```python
from build123d import *

# Parameters (mm, degrees)
F0_W     = 9.45931
F0_H     = 54.78517
F0_R     = 2.258507
F1_DEPTH = 0.4318
F0_R_2   = 1.35948
F2_DEPTH = 0.4064
F0_R_3   = 0.729172
F3_DEPTH = 0.3556
F4_DEPTH = 0.254


with BuildPart() as f1:
    # F0 (on Top) → F1 (new body, symmetric)
    with BuildSketch(Plane.XY):
        Rectangle(F0_W, F0_H)
        with Locations((0, -24.156982)):
            Circle(F0_R, mode=Mode.SUBTRACT)
    extrude(amount=F1_DEPTH, both=True)

    # F0 (on Top) → F2 (join)
    with BuildSketch(Plane.XY):
        with Locations((0, -24.156982)):
            Circle(F0_R)
        with Locations((0, -24.156982)):
            Circle(F0_R_2, mode=Mode.SUBTRACT)
    extrude(amount=F2_DEPTH)

    # F0 (on Top) → F3 (join)
    with BuildSketch(Plane.XY):
        with Locations((0, -24.156982)):
            Circle(F0_R_2)
        with Locations((0, -24.156982)):
            Circle(F0_R_3, mode=Mode.SUBTRACT)
    extrude(amount=F3_DEPTH)

    # F0 (on Top) → F4 (join)
    with BuildSketch(Plane.XY):
        with Locations((0, -24.156982)):
            Circle(F0_R_3)
    extrude(amount=F4_DEPTH)


solid = f1.part
```
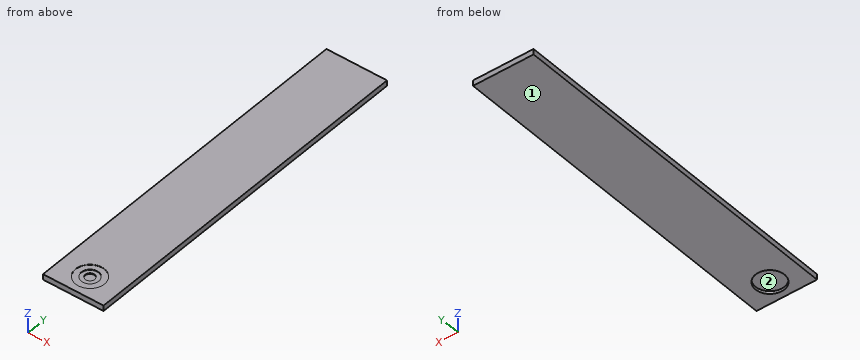
The listing builds one solid part. Answer for the finished solid, in the listing's coordinates (mm). Face numbers are marked on the shaded views. Round coordinates to 2 decimals unless told otherwise and drop trailing zeros. Write each loop counter-clockwise with the first axis right and the second up, starting at its lowest first coordinate (ties: lowest second). Pieces come first, ordered by that corner, then holes. Notation, with made-up numbers: (80, 47) -> (89, 47) arc R17 cw to (89, 70) -> close; hole circle Ø3 at (53.25, 68). An arc over 180 degrees is marked (long way). Answer as a JSON object with one key per item and string values. Group by question number.
Q1. Each of these flat-tipped pins is pushed along its axis until it touches: pin 1 Ø2.5 at (x, y) = (0, -25) entering from -Z; pin 2 Ø1.9 at (x, y) = (0, -24.16) entering from +Z. Where does it stop, or does it pass through?
Q2. Straight lines are drawn through the part: line 1 along Y through (x, z) = (0, -0.05); line 2 along Y through (x, z) = (0, 0.3). For each, find the intervals that lie inside material, in ascending order.
Q3. Section B-B (z = -0.3) is taken. Write down the section's boundary in (x, y), plus the area to 3 significant figures.
Q4. Determine the mould class of the marked faces 1 and 2 for opening direction Y: pulls with the +Y half, pulls with the -Y half, needs draft (parallel to the pull), parting line crosses it, or undercut.
Check values:
{
 "1": {"pin 1": "z = 0", "pin 2": "z = 0.36"},
 "2": {"line 1": "-27.39 to -26.42, -21.9 to 27.39", "line 2": "-27.39 to -24.89, -23.43 to 27.39"},
 "3": {"outline": "(-4.73, -27.39) -> (4.73, -27.39) -> (4.73, 27.39) -> (-4.73, 27.39) -> close; hole circle Ø4.52 at (0, -24.16)", "area": "502 mm^2"},
 "4": {"face 1": "needs draft", "face 2": "undercut"}
}
